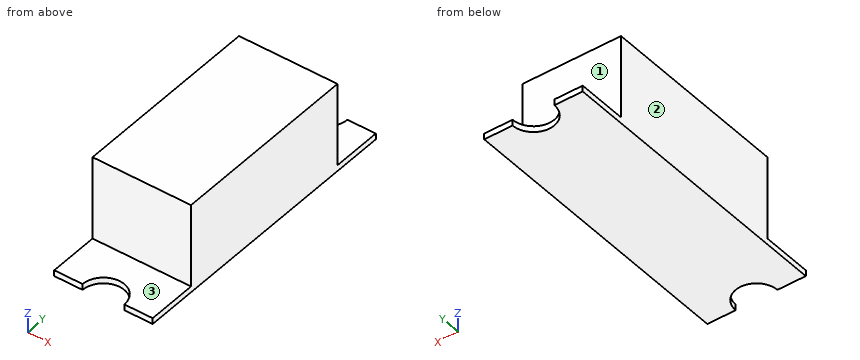
from build123d import *

# Parameters (mm, degrees)
ESQUISSE1_W        = 6.6
ESQUISSE1_H        = 12.8
BOSS_EXTRU_1_DEPTH = 5.6
ESQUISSE2_W        = 1.9
ESQUISSE2_H        = 12.8
ESQUISSE2_W_2      = 2.8
ESQUISSE2_H_2      = 3.35
BOSS_EXTRU_2_DEPTH = 0.4


with BuildPart() as part:
    # Esquisse1 → Boss.-Extru.1 (new body)
    with BuildSketch(Plane.XY):
        with Locations((-3.3, -6.4)):
            Rectangle(ESQUISSE1_W, ESQUISSE1_H)
    extrude(amount=BOSS_EXTRU_1_DEPTH)

    # Esquisse2 → Boss.-Extru.2 (add)
    with BuildSketch(Plane(origin=(0, 0, 0), x_dir=(-1, 0, 0), z_dir=(0, 0, -1))):
        with Locations((0.95, -6.4)):
            Rectangle(ESQUISSE2_W, ESQUISSE2_H)
        with Locations((3.3, -6.4)):
            Rectangle(ESQUISSE2_W_2, ESQUISSE2_H)
        with Locations((5.65, -6.4)):
            Rectangle(ESQUISSE2_W, ESQUISSE2_H)
        with Locations((0.95, -14.475)):
            Rectangle(ESQUISSE2_W, ESQUISSE2_H_2)
        with BuildLine():
            Line((4.7, -12.8), (1.9, -12.8))
            Line((1.9, -12.8), (1.9, -16.15))
            ThreePointArc((1.9, -16.15), (3.3, -14.75), (4.7, -16.15))
            Line((4.7, -16.15), (4.7, -12.8))
        make_face()
        with Locations((5.65, -14.475)):
            Rectangle(ESQUISSE2_W, ESQUISSE2_H_2)
        with Locations((0.95, 1.675)):
            Rectangle(ESQUISSE2_W, ESQUISSE2_H_2)
        with BuildLine():
            ThreePointArc((4.7, 3.35), (3.3, 1.95), (1.9, 3.35))
            Line((1.9, 3.35), (1.9, 0))
            Line((1.9, 0), (4.7, 0))
            Line((4.7, 0), (4.7, 3.35))
        make_face()
        with Locations((5.65, 1.675)):
            Rectangle(ESQUISSE2_W, ESQUISSE2_H_2)
    extrude(amount=BOSS_EXTRU_2_DEPTH)


solid = part.part
Model file for the job. Use its own axes, mm. Face numbers are marked on the shaded views. A direction names the side the tool comes from. Coordinates: 2 decimals unless noted, no trailing zeros. Order: outer loops, then holes, each group sorted by start corner. A loop starts at its lowest first (then second) coordinate and runs counter-clockwise, first axis right, second up. Notation, with made-up numbers: (-25, 52.5) -> (3, 52.5) arc R33 cw to (3, 84.5) -> close; hole circle Ø9 at (66, 21). An arc over 180 degrees is marked (long way). Return JSON: item names as keys, results as strings. Group by question number.
Item 1: Saw through at C-C on x = -3.3. Write the cut outline in (y, z), then the cut area to 3 significant figures.
Item 2: Saw through at A-A on x = -5.75. Write the cut outline in (y, z), then the cut area to 3 significant figures.
Item 3: Saw through at B-B on z = 0.45. Write the cut outline in (x, y), then the cut area to 3 significant figures.
Item 4: Tool access for the marked faces 1, 2 and 3: list every direction of +Z, -Z, +X, -X, +Y, -Y with a clear straight run to the whole face (end or side of a thin tool).
Item 5: Flat gauge pins, fed straight in: P1, Ø3.5, axis at x = -4, y = -14.5, coming from the +Z side; P2, Ø1.7, axis at x = -2, z = 3.5, coming from the -Y side; P3, Ø1.7, axis at x = -4.5, y = 2, coming from the +Z side. Where does each tip first touch, or does it go through?
Item 6: Wall check: line 1 along Y through (x, z) = (-2.5, 4.15); line 2 along Z through (x, y) = (-2.5, 1). Give the ranges that are in metal, low to high. Write a range as [from, to].
Values found:
{
 "1": {"outline": "(-14.75, -0.4) -> (1.95, -0.4) -> (1.95, 0) -> (0, 0) -> (0, 5.6) -> (-12.8, 5.6) -> (-12.8, 0) -> (-14.75, 0) -> close", "area": "78.4 mm2"},
 "2": {"outline": "(-16.15, -0.4) -> (3.35, -0.4) -> (3.35, 0) -> (0, 0) -> (0, 5.6) -> (-12.8, 5.6) -> (-12.8, 0) -> (-16.15, 0) -> close", "area": "79.5 mm2"},
 "3": {"outline": "(-6.6, -12.8) -> (0, -12.8) -> (0, 0) -> (-6.6, 0) -> close", "area": "84.5 mm2"},
 "4": {"face 1": "+Z, +X, -X, +Y", "face 2": "+Z, -Z, -X, +Y, -Y", "face 3": "+Z, +X, -X, -Y"},
 "5": {"P1": "stops at z = 5.6", "P2": "stops at y = -12.8", "P3": "stops at z = 0"},
 "6": {"line 1": "y = [-12.8, 0]", "line 2": "z = [-0.4, 0]"}
}
